Part model, mm, in its own coordinate system. A direction names the side the tool comes from. Give positions to 0.01 mm unless a question says otherwise; leave off trailing zeros. Order: outer loops, then holes, each group sorted by start corner. A loop starts at its lowest first (then second) coordinate and runs counter-clockwise, first axis right, second up. Notation, with made-up numbers: (20.5, -2) - (46.5, -2) arc R21 cw to (46.5, 16) - close; hole circle Ø1 at (5, 55). An arc over 180 degrees is marked (long way). Use a Markdown table: item, result. Add a question column.
from build123d import *

# Parameters (mm, degrees)
SKETCH1_R           = 0.95
BOSS_EXTRUDE1_DEPTH = 4
SKETCH2_W           = 16.2
SKETCH2_H           = 33.21
CUT_EXTRUDE2_DEPTH  = 2


with BuildPart() as part:
    # Sketch1 → Boss-Extrude1 (new body)
    with BuildSketch(Plane.XY):
        with BuildLine():
            Line((0, 26.21), (0, 7))
            Line((0, 7), (4, 7))
            Line((4, 7), (4, 5))
            Line((4, 5), (0, 5))
            Line((0, 5), (0, 2))
            ThreePointArc((0, 2), (0.585786438, 0.585786438), (2, 0))
            Line((2, 0), (14.2, 0))
            ThreePointArc((14.2, 0), (15.614213562, 0.585786438), (16.2, 2))
            Line((16.2, 2), (16.2, 5))
            Line((16.2, 5), (12.2, 5))
            Line((12.2, 5), (12.2, 7))
            Line((12.2, 7), (16.2, 7))
            Line((16.2, 7), (16.2, 26.21))
            Line((16.2, 26.21), (12.2, 26.21))
            Line((12.2, 26.21), (12.2, 28.21))
            Line((12.2, 28.21), (16.2, 28.21))
            Line((16.2, 28.21), (16.2, 31.21))
            ThreePointArc((16.2, 31.21), (15.614213562, 32.624213562), (14.2, 33.21))
            Line((14.2, 33.21), (2, 33.21))
            ThreePointArc((2, 33.21), (0.585786438, 32.624213562), (0, 31.21))
            Line((0, 31.21), (0, 28.21))
            Line((0, 28.21), (4, 28.21))
            Line((4, 28.21), (4, 26.21))
            Line((4, 26.21), (0, 26.21))
        make_face()
        with Locations((13.45, 2.5)):
            Circle(SKETCH1_R, mode=Mode.SUBTRACT)
        with Locations((10.2, 9.5)):
            Circle(SKETCH1_R, mode=Mode.SUBTRACT)
        with Locations((2.75, 30.71)):
            Circle(SKETCH1_R, mode=Mode.SUBTRACT)
        with Locations((6, 23.71)):
            Circle(SKETCH1_R, mode=Mode.SUBTRACT)
        with Locations((6, 9.5)):
            Circle(SKETCH1_R, mode=Mode.SUBTRACT)
        with Locations((2.75, 2.5)):
            Circle(SKETCH1_R, mode=Mode.SUBTRACT)
        with Locations((10.2, 23.71)):
            Circle(SKETCH1_R, mode=Mode.SUBTRACT)
        with Locations((13.45, 30.71)):
            Circle(SKETCH1_R, mode=Mode.SUBTRACT)
    extrude(amount=BOSS_EXTRUDE1_DEPTH)

    # Sketch2 → Cut-Extrude2 (cut)
    with BuildSketch(Plane.XY):
        with Locations((8.1, 16.605)):
            Rectangle(SKETCH2_W, SKETCH2_H)
    extrude(amount=CUT_EXTRUDE2_DEPTH, mode=Mode.SUBTRACT)


solid = part.part
1. Cut at C-C (y = 23.71). Write the cut outline in (x, z).
2. Cut at A-A (z = 3.55). State how many separate pieces and enclosed holes the cut face has, plus the area to 3 significant figures.
3. Cut at B-B (x = 10.2). Write the cut outline in (y, z).
4. Pin check, flat tip, straight feed: P1, Ø1.1, axis at x = 10.2, y = 23.71, coming from the +Z side. Stop position of the tip, or through.
5. Tool access for faces 1 (the face through (16.2, 30, 3)), 2 (the face through (2, 26.21, 3)), 3 (the face through (14, 5, 3)): list every direction of +Z, -Z, +X, -X, +Y, -Y with a clear straight run to the whole face (end or side of a thin tool).
6. Drill centre lines: probe 1 along Y at (x, z) = (10.2, 2.9); probe 2 along X at (y, z) = (30.71, 2.6); probe 3 along X at (y, z) = (23.71, 2.55). Where is each one in solid material? Low to high. Write a range as [from, to].
7. Mould opens along Y. For faces 4 (the face through (5.876, 10.442, 2.986)), 5 (the face through (0, 17, 3)), 6 (the face through (8, 33.21, 3)) say: released by +Y, released by -Y, zero draft, split by the parting line, or undercut.
Responses:
| question | item | result |
|---|---|---|
| 1 | outline | (0, 2) - (5.05, 2) - (5.05, 4) - (0, 4) - close; (6.95, 2) - (9.25, 2) - (9.25, 4) - (6.95, 4) - close; (11.15, 2) - (16.2, 2) - (16.2, 4) - (11.15, 4) - close |
| 2 | separate pieces | 1 |
| 2 | enclosed holes | 8 |
| 2 | area | 480 mm² |
| 3 | outline | (0, 2) - (8.55, 2) - (8.55, 4) - (0, 4) - close; (10.45, 2) - (22.76, 2) - (22.76, 4) - (10.45, 4) - close; (24.66, 2) - (33.21, 2) - (33.21, 4) - (24.66, 4) - close |
| 4 | P1 | passes through |
| 5 | face 1 | +Z, -Z, +X, +Y, -Y |
| 5 | face 2 | +Z, -Z, -X |
| 5 | face 3 | +Z, -Z, +X |
| 6 | probe 1 | y = [0, 8.55], [10.45, 22.76], [24.66, 33.21] |
| 6 | probe 2 | x = [0, 1.8], [3.7, 12.5], [14.4, 16.2] |
| 6 | probe 3 | x = [0, 5.05], [6.95, 9.25], [11.15, 16.2] |
| 7 | face 4 | undercut |
| 7 | face 5 | zero draft |
| 7 | face 6 | released by +Y |
